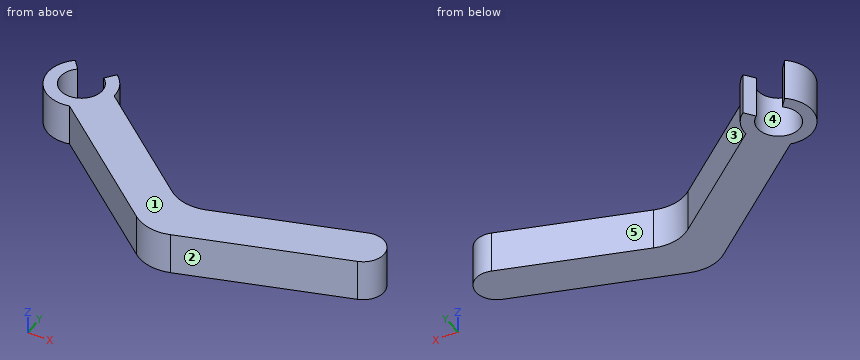
Autodesk Inventor part; units mm, degrees
ref_plane "YZ Plane" through (0, 0, 0) normal (1, 0, 0) x (0, 1, 0)
ref_plane "XZ Plane" through (0, 0, 0) normal (0, 1, 0) x (-1, 0, 0)
ref_plane "XY Plane" through (0, 0, 0) normal (0, 0, 1) x (1, 0, 0)
sketch "Sketch1" plane through (0, 0, 0) normal (0, 0, 1) x (1, 0, 0)
  line L0 (7.0984, -37.2544) -> (-17.2546, -44.4717)
  line L1 (-19.0349, -38.4646) -> (5.3181, -31.2472)
  arc A0 (7.0984, -37.2544) -> (5.3181, -31.2472) centre (6.2488, -34.2388) ccw
  line L2 (-42.5288, -26.9478) -> (-20.5002, -45.4336)
  line L3 (-20.5002, -45.4336) -> (-17.2546, -44.4717)
  line L4 (-38.4744, -22.1514) -> (-19.0349, -38.4646)
  line L5 (-40.3781, -18.0047) -> (-41.5692, -19.4938)
  line L6 (-45.5333, -19.4938) -> (-46.7244, -18.0047)
  arc A1 (-45.5333, -19.4938) -> (-41.5692, -19.4938) centre (-43.5513, -21.9717) ccw
  arc A2 (-46.7244, -18.0047) -> (-42.5288, -26.9478) centre (-43.5513, -21.9717) ccw
  arc A3 (-38.4744, -22.1514) -> (-40.3781, -18.0047) centre (-43.5513, -21.9717) ccw
  point P0 (0, 0)
  point P1 (0, 0)
extrude "Extrusion1" add sketch "Sketch1" along normal blind 6.35
fillet "Fillet1" radius 6.35 2 edges at (-20.5002, -45.4336, 3.175) (-19.0349, -38.4646, 3.175)
properties part number "Holder left arm"
Can you work these out from the model? Positions are in its coordinate system, mm. Face numbers are marked on the shaded views. A direction names the side the tool comes from. Coordinates: 2 decimals unless noted, no trailing zeros. Loops run counter-clockwise (first coordinate to the right, second up) from the corner with the lowest first, then second, coordinate; pieces in that order, holes last.
1) Imagine slicing it at A-A on y = -23.25. List the corners of the cut face in (x, z) for me, plus the area to 3 significant figures.
2) I need wall thicknesses on probe 1 along X at (y, z) = (-23.75, 6.25); probe 2 along X at (y, z) = (-24.25, 2); probe 3 along X at (y, z) = (-25.5, 1.25). Which ranges of each line are inside material? Lowest first, please.
3) For pin 1 (1.5 mm diameter, centred on x = -31.5, y = -28.5, fed in from -Z); pin 2 (2 mm diameter, centred on y = -39.5, z = 2, fed in from -X); pin 3 (1.5 mm diameter, centred on x = -13.5, z = 5, fed in from +Y); pin 4 (1 mm diameter, centred on x = -3.5, z = 2.5, fed in from -Y), each with a flat end and sliding along its axis, tell me the tip position at first contact or that it passes through.
4) Thinking about a two-plate mould opening in X: for the marked faces 1, 2 and 3, which applies, pulls with the +X half, pulls with the -X half, needs draft (parallel to the pull), parting line crosses it, or undercut?
5) Imagine slicing it at C-C on x = -28.5. List the corners of the cut face in (y, z) for me.
6) Imagine slicing it at D-D on y = -38.75. List the corners of the cut face in (x, z) for me.
7) Imagine slicing it at B-B on y = -35. List the corners of the cut face in (x, z) for me.
8) Which directions (+Z, -Z, +X, -X, +Y, -Y) give clear straight access to the entire face, cutting with the end or side of a thin tool? Please do the marked faces 4 and 5.
Completed:
1. outline: (-48.47, 0) - (-46.46, 0) - (-46.46, 6.35) - (-48.47, 6.35) - close; (-40.65, 0) - (-37.17, 0) - (-37.17, 6.35) - (-40.65, 6.35) - close
1. area: 34.9 mm2
2. probe 1: x = -48.31 to -46.18, -40.92 to -36.57
2. probe 2: x = -48.09 to -45.76, -41.34 to -35.97
2. probe 3: x = -47.21 to -34.48
3. pin 1: stops at z = 0
3. pin 2: stops at x = -28.76
3. pin 3: stops at y = -36.6
3. pin 4: stops at y = -40.54
4. face 1: needs draft
4. face 2: pulls with the +X half
4. face 3: undercut
5. outline: (-38.72, 0) - (-30.52, 0) - (-30.52, 6.35) - (-38.72, 6.35) - close
6. outline: (-28.46, 0) - (2.05, 0) - (2.05, 6.35) - (-28.46, 6.35) - close
7. outline: (-32.93, 0) - (-23.16, 0) - (-23.16, 6.35) - (-32.93, 6.35) - close; (-7.34, 0) - (9.29, 0) - (9.29, 6.35) - (-7.34, 6.35) - close
8. face 4: +Z, -Z
8. face 5: +Z, -Z, +Y
